Part model, mm, in its own coordinate system. Round coordinates to 2 decimals unless told otherwise and drop trailing zeros. Write each loop counter-clockwise with the first axis right and the second up, starting at its lowest first coordinate (ties: lowest second). Pieces come first, ordered by that corner, then holes. Notation, with made-up numbers: (74, 0) -> (98, 0) arc R15 ccw to (98, 11) -> close; hole circle Ø3 at (-8, 17.25). An arc over 180 degrees is marked (long way). Return JSON: item names as keys, results as strings. Group by question number.
(1) Saw through at A-A (x = 0). List the corners of the cut face in (y, z), plus the area to 3 significant figures.
(2) Drop flat-ended pins along their axis: pin 1 Ø1.3 at (x, z) = (1.5, 3) entering from -Y; pin 2 Ø1 at (x, z) = (1, 1.5) entering from +Y (3 decimals). Give the stop position or say it passes through.
(3) Saw through at B-B (z = 3.1). List the corners of the cut face in (x, y).
(4) Drill centre lines: L1, parallel to Y at x = 0, z = 3; L2, parallel to Y at x = -0.5, z = 1.25 (3 decimals); L3, parallel to X at y = 13, z = 1.6. Where is each one in solid material? Low to high. Write a range as from..to.
(5) Saw through at D-D (x = -13). List the corners of the cut face in (y, z).
(6) Saw through at C-C (x = -19). List the corners of the cut face in (y, z).
from build123d import *

# Parameters (mm, degrees)
SKETCH1_W           = 15
SKETCH1_H           = 10
SKETCH1_H_2         = 7.5
BOSS_EXTRUDE1_DEPTH = 4.5
SKETCH2_R           = 2.5
CUT_EXTRUDE1_DEPTH  = 10


with BuildPart() as part:
    # Sketch1 → Boss-Extrude1 (new body)
    with BuildSketch(Plane.XY):
        Polygon((-25, -55), (-10, -55), (10, -55), (25, -55), (25, 5), (-25, 5), align=None)
        with Locations((17.5, -60)):
            Rectangle(SKETCH1_W, SKETCH1_H)
        with Locations((-17.5, -60)):
            Rectangle(SKETCH1_W, SKETCH1_H)
        with BuildLine():
            Line((-25, 5), (25, 5))
            ThreePointArc((25, 5), (0, 30), (-25, 5))
        make_face()
        with Locations((-17.5, -68.75)):
            Rectangle(SKETCH1_W, SKETCH1_H_2)
        with Locations((17.5, -68.75)):
            Rectangle(SKETCH1_W, SKETCH1_H_2)
    extrude(amount=BOSS_EXTRUDE1_DEPTH)

    # Sketch2 → Cut-Extrude1 (cut)
    with BuildSketch(Plane.XY.offset(4.5)):
        with Locations((0, 10)):
            Circle(SKETCH2_R)
    extrude(amount=-CUT_EXTRUDE1_DEPTH, mode=Mode.SUBTRACT)


solid = part.part
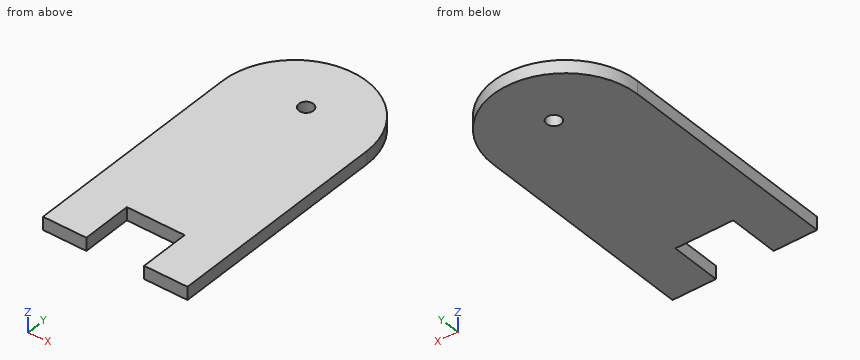
Computed values:
{
 "1": {"outline": "(-55, 0) -> (7.5, 0) -> (7.5, 4.5) -> (-55, 4.5) -> close; (12.5, 0) -> (30, 0) -> (30, 4.5) -> (12.5, 4.5) -> close", "area": "360 mm2"},
 "2": {"pin 1": "y = -55", "pin 2": "y = 29.995"},
 "3": {"outline": "(-25, -72.5) -> (-10, -72.5) -> (-10, -55) -> (10, -55) -> (10, -72.5) -> (25, -72.5) -> (25, 5) arc R25 ccw to (-25, 5) -> close; hole circle Ø5 at (0, 10)"},
 "4": {"L1": "-55..7.5, 12.5..30", "L2": "-55..7.551, 12.449..29.995", "L3": "-23.69..23.69"},
 "5": {"outline": "(-72.5, 0) -> (26.35, 0) -> (26.35, 4.5) -> (-72.5, 4.5) -> close"},
 "6": {"outline": "(-72.5, 0) -> (21.25, 0) -> (21.25, 4.5) -> (-72.5, 4.5) -> close"}
}
